Model file for the job. Use its own axes, mm. Face numbers are marked on the shaded views. A direction names the side the tool comes from. Round coordinates to 2 decimals unless told otherwise and drop trailing zeros. Order: outer loops, then holes, each group sorted by start corner. A loop starts at its lowest first (then second) coordinate and runs counter-clockwise, first axis right, second up. Notation, with made-up numbers: (-2, -3) - (47, -3) arc R34 cw to (47, 30) - close; hole circle Ø2 at (-26, 65). An arc over 180 degrees is marked (long way). Use one line per item in the form item = value.
from build123d import *

# Parameters (mm, degrees)
SZKIC1_W                                             = 400
SZKIC1_H                                             = 420
DODANIE_WYCI_GNI_CIE1_DEPTH                          = 14
POG_BIENIE_WALCOWE_POD_M5_WKR_T_DO_CZ_CI_D           = 5.5
POG_BIENIE_WALCOWE_POD_M5_WKR_T_DO_CZ_CI_CBORE_D     = 9
POG_BIENIE_WALCOWE_POD_M5_WKR_T_DO_CZ_CI_CBORE_DEPTH = 6
SZKIC10_W                                            = 70
SZKIC10_H                                            = 4
WYTNIJ_WYCI_GNI_CIE1_DEPTH                           = 50
ZAOKR_GLENIE1_R                                      = 10
SKETCH_1_R                                           = 4.5
CUT_EXTRUDE_1_DEPTH                                  = 6
SKETCH_2_R                                           = 2.75
CUT_EXTRUDE_2_DEPTH                                  = 291.337734372
EXTRUDE_2_DEPTH                                      = 25
FILLET_3_R                                           = 10
FILLET_4_R                                           = 10
SKETCH_5_R                                           = 3.5
CUT_EXTRUDE_3_DEPTH                                  = 292.075591557


with BuildPart() as part:
    # Szkic1 → Dodanie-wyciągnięcie1 (new body)
    with BuildSketch(Plane(origin=(0, 0, 0), x_dir=(1, 0, 0), z_dir=(0, 1, 0))):
        Rectangle(SZKIC1_W, SZKIC1_H)
    extrude(amount=DODANIE_WYCI_GNI_CIE1_DEPTH)

    # Pogłębienie walcowe pod M5 Wkręt do części metalowych z łbem sześciokątnym1 (through all)
    with Locations(Plane(origin=(0, 14, 0), x_dir=(1, 0, 0), z_dir=(0, 1, 0))):
        with Locations((-87.5, -141), (-87.5, -109), (-57.5, -141), (-57.5, -109), (57.5, -141), (57.5, -109), (87.5, -109), (87.5, -141)):
            pog_bienie_walcowe_pod_m5_wkr_t_do_cz_ci = CounterBoreHole(POG_BIENIE_WALCOWE_POD_M5_WKR_T_DO_CZ_CI_D / 2, POG_BIENIE_WALCOWE_POD_M5_WKR_T_DO_CZ_CI_CBORE_D / 2, POG_BIENIE_WALCOWE_POD_M5_WKR_T_DO_CZ_CI_CBORE_DEPTH)

    # Lustro3: Pogłębienie walcowe pod M5 Wkręt do części metalowych z łbem sześciokątnym1 across plane
    add(pog_bienie_walcowe_pod_m5_wkr_t_do_cz_ci.mirror(Plane.XY), mode=Mode.SUBTRACT)

    # Szkic10 → Wytnij-wyciągnięcie1 (cut)
    with BuildSketch(Plane.ZY.offset(200)):
        with Locations((0, 2)):
            Rectangle(SZKIC10_W, SZKIC10_H)
    extrude(amount=-WYTNIJ_WYCI_GNI_CIE1_DEPTH, mode=Mode.SUBTRACT)

    # Zaokrąglenie1
    zaokr_glenie1_edges = [part.edges().sort_by_distance(p)[0] for p in [
        (-150, 2, -35),
        (-150, 2, 35),
    ]]
    fillet(zaokr_glenie1_edges, radius=ZAOKR_GLENIE1_R)

    # 草图1 → 切除-拉伸1 (cut)
    with BuildSketch(Plane(origin=(0, 14, 0), x_dir=(1, 0, 0), z_dir=(0, 1, 0))):
        with Locations(Location((11.5, 32, 0), (0, 0, 270))):
            Circle(SKETCH_1_R)
        with Locations(Location((-11.5, 32, 0), (0, 0, 90))):
            Circle(SKETCH_1_R)
        with Locations(Location((-11.5, -32, 0), (0, 0, 270))):
            Circle(SKETCH_1_R)
        with Locations(Location((11.5, -32, 0), (0, 0, 90))):
            Circle(SKETCH_1_R)
    extrude(amount=-CUT_EXTRUDE_1_DEPTH, mode=Mode.SUBTRACT)

    # 草图2 → 切除-拉伸2 (cut, through all)
    with BuildSketch(Plane(origin=(0, 14, 0), x_dir=(1, 0, 0), z_dir=(0, 1, 0))):
        with Locations(Location((11.5, 32, 0), (0, 0, 270))):
            Circle(SKETCH_2_R)
        with Locations(Location((-11.5, 32, 0), (0, 0, 90))):
            Circle(SKETCH_2_R)
        with Locations(Location((-11.5, -32, 0), (0, 0, 270))):
            Circle(SKETCH_2_R)
        with Locations(Location((11.5, -32, 0), (0, 0, 90))):
            Circle(SKETCH_2_R)
    extrude(amount=-CUT_EXTRUDE_2_DEPTH, mode=Mode.SUBTRACT)

    # 草图4 → 凸台-拉伸2 (add)
    with BuildSketch(Plane(origin=(0, 14, 0), x_dir=(1, 0, 0), z_dir=(0, 1, 0))):
        Polygon((-200, 210), (-200, -210), (200, -210), (200, -175), (-165, -175), (-165, 210), align=None)
    extrude(amount=EXTRUDE_2_DEPTH)

    # 圆角3
    fillet_3_edges = [part.edges().sort_by_distance(p)[0] for p in [
        (200, 39, 192.5),
    ]]
    fillet(fillet_3_edges, radius=FILLET_3_R)

    # 圆角4
    fillet_4_edges = [part.edges().sort_by_distance(p)[0] for p in [
        (-182.5, 39, -210),
    ]]
    fillet(fillet_4_edges, radius=FILLET_4_R)

    # 草图5 → 切除-拉伸3 (cut, through all)
    with BuildSketch(Plane(origin=(0, 14, 0), x_dir=(1, 0, 0), z_dir=(0, 1, 0))):
        with Locations(Location((100, -65, 0), (0, 0, 270))):
            Circle(SKETCH_5_R)
        with Locations(Location((180, -65, 0), (0, 0, 270))):
            Circle(SKETCH_5_R)
        with Locations(Location((180, -25, 0), (0, 0, 90))):
            Circle(SKETCH_5_R)
        with Locations(Location((100, -25, 0), (0, 0, 90))):
            Circle(SKETCH_5_R)
        with Locations(Location((5, 110, 0), (0, 0, 270))):
            Circle(SKETCH_5_R)
        with Locations(Location((5, 190, 0), (0, 0, 270))):
            Circle(SKETCH_5_R)
        with Locations(Location((-35, 190, 0), (0, 0, 90))):
            Circle(SKETCH_5_R)
        with Locations(Location((-35, 110, 0), (0, 0, 90))):
            Circle(SKETCH_5_R)
    extrude(amount=-CUT_EXTRUDE_3_DEPTH, mode=Mode.SUBTRACT)


solid = part.part
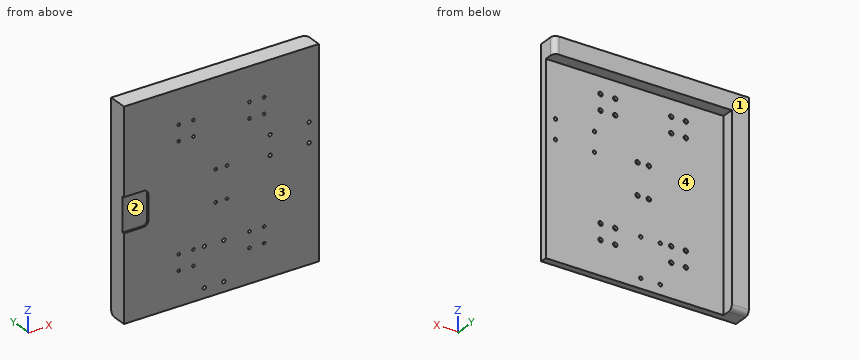
(1) Slice it at A-A on z = -10. Give the cut face in (x, y).
Report:
outline = (-200, 4) - (-150, 4) - (-150, 0) - (200, 0) - (200, 14) - (-165, 14) - (-165, 39) - (-200, 39) - close
(2) Pull direction Z, two halves, no side cores. Call the marked faces 1 and 2: released by +Z, released by -Z, zero draft, split by the parting line, or undercut.
Report:
face_1 = zero draft
face_2 = undercut
(3) Tool access for the marked faces 3 and 4: list every direction of +Z, -Z, +X, -X, +Y, -Y with a clear straight run to the whole face (end or side of a thin tool).
Report:
face_3 = +Z, -Z, +X, -X, -Y
face_4 = -Z, +X, +Y
(4) Pin check, flat tips, straight feed: pin 1 (8 mm diameter, centred on x = -148, z = 150.5, fed in from +Y); pin 2 (1.5 mm diameter, centred on y = 30.5, z = 119, fed in from +X); pin 3 (2.5 mm diameter, centred on x = -59, z = -108.5, fed in from +Y); pin 4 (4 mm diameter, centred on x = 180, z = 65, fed in from -Y). Stop position of each tip, or through.
Report:
pin_1 = 14
pin_2 = -165
pin_3 = 8
pin_4 = through
(5) Probe probe 1 along X at (y, z) = (5, 109); probe 2 along Z at (x, y) = (-57, 3); probe 3 along Z at (x, y) = (-57, 12). List the from-to ranges inside material, lowest first. Write a range as [from, to].
Report:
probe_1 = [-200, -90.25], [-84.75, -60.25], [-54.75, 54.75], [60.25, 84.75], [90.25, 200]
probe_2 = [-210, -143.7], [-138.3, -111.7], [-106.3, 106.3], [111.7, 138.3], [143.7, 210]
probe_3 = [-210, -145.47], [-136.53, -113.47], [-104.53, 104.53], [113.47, 136.53], [145.47, 210]
(6) Slice it at B-B on y = 22.5. Give the cut face in (x, z), then the cut area to 3 significant figures.
Report:
outline = (-200, -210) - (-165, -210) - (-165, 175) - (200, 175) - (200, 210) - (-200, 210) - close
area = 27,500 mm2
(7) Slice it at C-C on x = -47. Give the cut face in (y, z).
Report:
outline = (0, -210) - (14, -210) - (14, 175) - (39, 175) - (39, 210) - (0, 210) - close
